Here's how the part is built. I have some questions about the finished solid (model axes, mm). Face numbers are marked on the shaded views. Coordinates: 2 decimals unless noted, no trailing zeros. Order: outer loops, then holes, each group sorted by start corner. A loop starts at its lowest first (then second) coordinate and runs counter-clockwise, first axis right, second up. Notation, with made-up numbers: (-12, -27) - (35, -27) arc R17 cw to (35, -19) - close; hole circle Ø1 at (-5, 40.5). An arc over 180 degrees is marked (long way). Use one line per item in the form item = value. Start each with the question number.
from build123d import *

# Parameters (mm, degrees)
PAD_DEPTH       = 20
SKETCH001_R     = 3
PAD001_DEPTH    = 5
SKETCH002_R     = 1.35
POCKET_DEPTH    = 14.7989589711
SKETCH003_R     = 1.4
POCKET001_DEPTH = 13.8999794856
SKETCH004_R     = 3
SKETCH004_R_2   = 1.6
PAD002_DEPTH    = 4
SKETCH005_R     = 3
SKETCH005_R_2   = 1.6
PAD003_DEPTH    = 8


with BuildPart() as part:
    # Sketch → Pad (new body, symmetric)
    with BuildSketch(Plane.XY):
        Polygon((0, 0), (-48.9897948557, 10), (-48.9897948557, 0), align=None)
    extrude(amount=PAD_DEPTH, both=True)

    # Sketch001 (on Face1 of Pad) → Pad001 (join)
    with BuildSketch(Plane(origin=(0, 0, 0), x_dir=(-0.9797958971, 0.2, 0), z_dir=(0.2, 0.9797958971, 0))):
        with Locations((42, 15.5)):
            Circle(SKETCH001_R)
        with Locations((42, -15.5)):
            Circle(SKETCH001_R)
        with Locations((11, -15.5)):
            Circle(SKETCH001_R)
        with Locations((11, 15.5)):
            Circle(SKETCH001_R)
    extrude(amount=PAD001_DEPTH)

    # Sketch002 (on Face11 of Pad001) → Pocket (cut, through all)
    with BuildSketch(Plane(origin=(1, 4.8989794856, 0), x_dir=(-0.9797958971, 0.2, 0), z_dir=(0.2, 0.9797958971, 0))):
        with Locations((42, -15.5)):
            Circle(SKETCH002_R)
        with Locations((11, -15.5)):
            Circle(SKETCH002_R)
        with Locations((42, 15.5)):
            Circle(SKETCH002_R)
        with Locations((11, 15.5)):
            Circle(SKETCH002_R)
    extrude(amount=-POCKET_DEPTH, mode=Mode.SUBTRACT)

    # Sketch003 (on Face2 of Pocket) → Pocket001 (cut, through all)
    with BuildSketch(Plane.XZ):
        with Locations((-15, 0)):
            Circle(SKETCH003_R)
        with Locations((-33.9897948557, 0)):
            Circle(SKETCH003_R)
    extrude(amount=-POCKET001_DEPTH, mode=Mode.SUBTRACT)

    # Sketch004 (on Face2 of Pocket001) → Pad002 (join)
    with BuildSketch(Plane.XZ):
        with Locations((-15, 0)):
            Circle(SKETCH004_R)
        with Locations((-15, 0)):
            Circle(SKETCH004_R_2, mode=Mode.SUBTRACT)
    extrude(amount=-PAD002_DEPTH)

    # Sketch005 (on Face2 of Pad002) → Pad003 (join)
    with BuildSketch(Plane.XZ):
        with Locations((-33.9897948557, 0)):
            Circle(SKETCH005_R)
        with Locations((-33.9897948557, 0)):
            Circle(SKETCH005_R_2, mode=Mode.SUBTRACT)
    extrude(amount=-PAD003_DEPTH)


solid = part.part
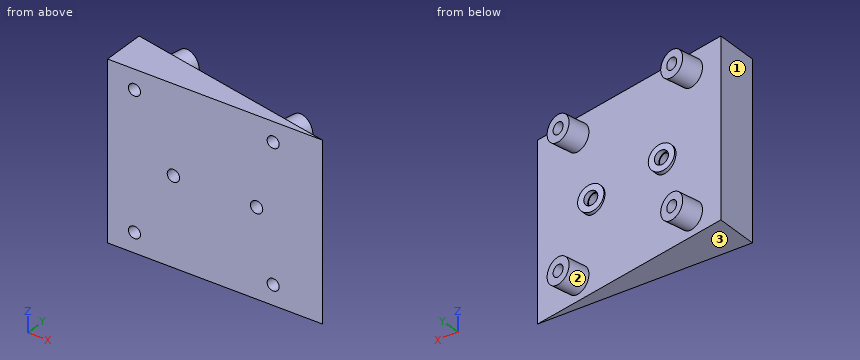
1) Suppose I cut it at A-A, the plane z = 0. List the corners of the cut face in (x, y) for me, then the cut area to 3 significant figures.
2) Suppose I cut it at D-D, the plane y = 11.5. Give the number of separate pieces and of enclosed holes in the cut face, then the cut area to 3 significant figures.
3) I need wall thicknesses on probe 1 along Z at (x, y) = (-38.5, 8); probe 2 along Z at (x, y) = (-15, 1); probe 3 along Z at (x, y) = (-41, 5.5). Which ranges of each line are inside material? Lowest first, please. Write a range as [from, to].
4) If we mould it in two halves opening along X, with no side actions, what happens to the marked faces 1, 2 and 3? For each: pulls with the +X half, pulls with the -X half, needs draft (parallel to the pull), parting line crosses it, or undercut.
5) Suppose I cut it at C-C, the plane z = 4. List the corners of the cut face in (x, y) for me, then the cut area to 3 significant figures.
6) Suppose I cut it at B-B, the plane x = -14.5. List the corners of the cut face in (y, z) for me.
7) For pin 1 (5 mm diameter, centred on x = -15, z = 0, fed in from +Y); pin 2 (3.5 mm diameter, centred on x = -33.99, z = 0, fed in from -Y); pin 3 (8 mm diameter, centred on x = -8, z = 14, fed in from +Y); pin 4 (4 mm diameter, centred on x = -33.99, z = 0, fed in from +Y), each with a flat end and sliding along its axis, tell me the tip position at first contact or that it passes through.
From the geometry:
q1.outline = (-48.99, 0) - (-35.39, 0) - (-35.39, 7.22) - (-35.59, 7.26) - (-35.59, 8) - (-36.99, 8) - (-36.99, 7.55) - (-48.99, 10) - close; (-32.59, 0) - (-16.4, 0) - (-16.4, 3.35) - (-16.6, 3.39) - (-16.6, 4) - (-18, 4) - (-18, 3.67) - (-30.99, 6.33) - (-30.99, 8) - (-32.39, 8) - (-32.39, 6.61) - (-32.59, 6.65) - close; (-13.6, 0) - (0, 0) - (-12, 2.45) - (-12, 4) - (-13.4, 4) - (-13.4, 2.74) - (-13.6, 2.78) - close
q1.area = 223 mm2
q2.separate_pieces = 2
q2.enclosed_holes = 2
q2.area = 46.0 mm2
q3.probe_1 = [-16.85, -14.15], [14.15, 16.85]
q3.probe_2 = [-20, -1.4], [1.4, 20]
q3.probe_3 = [-20, -16.64], [-14.36, 14.36], [16.64, 20]
q4.face_1 = pulls with the -X half
q4.face_2 = undercut
q4.face_3 = needs draft
q5.outline = (-48.99, 0) - (0, 0) - (-48.99, 10) - close
q5.area = 245 mm2
q6.outline = (0, -20) - (2.96, -20) - (2.96, -2.96) - (4, -2.96) - (4, -1.52) - (2.96, -1.52) - (2.96, -1.31) - (0, -1.31) - close; (0, 1.31) - (2.96, 1.31) - (2.96, 1.52) - (4, 1.52) - (4, 2.96) - (2.96, 2.96) - (2.96, 20) - (0, 20) - close
q7.pin_1 = 4
q7.pin_2 = 0
q7.pin_3 = 7.55
q7.pin_4 = 8
